Read the model definition and answer for the solid it produces. Units are mm, in the model's axes. A direction names the side the tool comes from. Coordinates: 2 decimals unless noted, no trailing zeros. Write each loop counter-clockwise with the first axis right and the second up, starting at its lowest first coordinate (ties: lowest second). Pieces come first, ordered by that corner, then holes.
Item 1: Section C-C (y = 6.5) is taken. Give the vertices of the cut face in (x, z), then the cut area to 3 significant figures.
Item 2: Determine the mould class of faces 1 (the face through (2.5, 1, -22.5)), 2 (the face through (2, -1, -5)), 3 (the face through (2, 0, -2)) for opening direction Z: released by +Z, released by -Z, zero draft, split by the parting line, or undercut.
Item 3: Each of these flat-tipped pins is pushed along its axis until it touches: P1, Ø2, axis at x = 1, z = -18, coming from the -Y side; P2, Ø1.6, axis at x = 3, y = -1, coming from the -Z side; P3, Ø1.5, axis at x = 2, z = -11, coming from the +Y side; P4, Ø2.5, axis at y = 7, z = -23, coming from the -X side. Where does it stop, or does it pass through?
Item 4: Section D-D (z = -23) is taken. Give the vertices of the cut face in (x, y).
Item 5: A tool of negligible diameter and unlimited length cuts with its end or side. For faces 4 (the face through (2, -2, -6)), 5 (the face through (0, 5, -13)), 6 (the face through (2, 0, -25)), 7 (the face through (0.76, 7.676, -25.146)), 8 (the face through (2, -1, -7)), from which of +Z, -Z, +X, -X, +Y, -Y can it reach the whole face along a straight path? Write none if from no direction.
Item 6: Section B-B (x = 0.55) is taken. Give the vertices of the cut face in (y, z), then the cut area to 3 significant figures.
Item 7: Section A-A (y = -0.5) is taken. Give the vertices of the cut face in (x, z).
Item 8: Straight lines are drawn through the part: probe 1 along Y at (x, z) = (3.3, -14); probe 2 along Z at (x, y) = (1.15, 0.75); probe 3 along Z at (x, y) = (1.1, 5). For each, find the intervals that lie inside material, in ascending order.
from build123d import *

# Parameters (mm, degrees)
BASE_W                    = 5
BASE_H                    = 26.5
BODY_DEPTH                = 11.5
F_6_0MM_MOTOR_D           = 6
F_3_0MM_BEARINGS_D        = 3
WEIGHT_SAVER_REACH        = 31.317
SKETCH9_W                 = 18.15
SKETCH9_H                 = 1.5
FILLET2_R                 = 3
FILLET1_R                 = 4
FILLET4_R                 = 4
FILLET5_R                 = 4
SKETCH10_W                = 5
SKETCH10_H                = 2
MOUNTING_DEPTH            = 2
MOUNTIN_UNDERCUT_REACH    = 31.317
F_4_0MM_DOWEL_HOLE2_D     = 4.5
F_4_0MM_DOWEL_HOLE2_DEPTH = 1.5


with BuildPart() as part:
    # base → body (new body)
    with BuildSketch(Plane(origin=(0, 0, 0), x_dir=(1, 0, 0), z_dir=(0, 1, 0))):
        with Locations((2.5, 13.25)):
            Rectangle(BASE_W, BASE_H)
    extrude(amount=BODY_DEPTH)

    # Ø6.0mm motor (through all)
    with Locations(Plane(origin=(5, 0, 0), x_dir=(0, 0, -1), z_dir=(1, 0, 0))):
        with Locations((5, 7)):
            Hole(F_6_0MM_MOTOR_D / 2)

    # Ø3.0mm bearings (through all)
    with Locations(Plane(origin=(5, 0, 0), x_dir=(0, 0, -1), z_dir=(1, 0, 0))):
        with Locations((14, 7), (23, 7)):
            Hole(F_3_0MM_BEARINGS_D / 2)

    # Sketch9 → weight_saver (cut, up to next)
    with BuildSketch(Plane(origin=(5, 0, 0), x_dir=(0, 0, -1), z_dir=(1, 0, 0)), mode=Mode.PRIVATE) as weight_saver_sk1:
        with Locations((17.425, 10.75)):
            Rectangle(SKETCH9_W, SKETCH9_H)
    weight_saver_tool1 = extrude(weight_saver_sk1.sketch, amount=-WEIGHT_SAVER_REACH, mode=Mode.PRIVATE) & part.part
    add(weight_saver_tool1.solids().sort_by_distance((5, 10.75, -17.425))[0], mode=Mode.SUBTRACT)

    # Fillet2
    fillet2_edges = [part.edges().sort_by_distance(p)[0] for p in [
        (2.5, 10, -26.5),
    ]]
    fillet(fillet2_edges, radius=FILLET2_R)

    # Fillet1
    fillet1_edges = [part.edges().sort_by_distance(p)[0] for p in [
        (2.5, 11.5, 0),
    ]]
    fillet(fillet1_edges, radius=FILLET1_R)

    # Fillet4
    # the kernel refuses this fillet: 4 mm, written as the material it adds along each edge
    with BuildSketch(Plane(origin=(5, 10, -8.35), x_dir=(0, 1, 0), z_dir=(-1, 0, 0))) as fillet4_piece_1:
        with BuildLine():
            CenterArc((4, 3.122498999), FILLET4_R, 180, 51.317812547)
            Line((0, 3.122498999), (-0.08, 3.122498999))
            Line((-0.08, 3.122498999), (-0.08, 0))
            Line((-0.08, 0), (0, -0.08))
            ThreePointArc((0, -0.08), (0.75, -0.08), (1.45, -0.06244998))
            Line((1.45, -0.06244998), (1.5, 0))
        make_face()
    extrude(amount=5)

    # Fillet5
    fillet5_edges = [part.edges().sort_by_distance(p)[0] for p in [
        (2.5, 11.5, -8.35),
    ]]
    fillet(fillet5_edges, radius=FILLET5_R)

    # Sketch10 → mounting (add)
    with BuildSketch(Plane.XZ):
        with Locations((2.5, -6)):
            Rectangle(SKETCH10_W, SKETCH10_H)
        with Locations((2.5, -20.5)):
            Rectangle(SKETCH10_W, SKETCH10_H)
    extrude(amount=MOUNTING_DEPTH)

    # mounting_undercut → mountin_undercut (cut, up to next)
    with BuildSketch(Plane(origin=(5, 0, 0), x_dir=(0, 0, -1), z_dir=(1, 0, 0)), mode=Mode.PRIVATE) as mountin_undercut_sk1:
        with BuildLine():
            Line((3, 0), (5, 0))
            ThreePointArc((5, 0), (4, 1), (3, 0))
        make_face()
    mountin_undercut_tool1 = extrude(mountin_undercut_sk1.sketch, amount=-MOUNTIN_UNDERCUT_REACH, mode=Mode.PRIVATE) & part.part
    # mounting_undercut → mountin_undercut (cut, up to next)
    with BuildSketch(Plane(origin=(5, 0, 0), x_dir=(0, 0, -1), z_dir=(1, 0, 0)), mode=Mode.PRIVATE) as mountin_undercut_sk2:
        with BuildLine():
            Line((7, 0), (9, 0))
            ThreePointArc((9, 0), (8, 1), (7, 0))
        make_face()
    mountin_undercut_tool2 = extrude(mountin_undercut_sk2.sketch, amount=-MOUNTIN_UNDERCUT_REACH, mode=Mode.PRIVATE) & part.part
    # mounting_undercut → mountin_undercut (cut, up to next)
    with BuildSketch(Plane(origin=(5, 0, 0), x_dir=(0, 0, -1), z_dir=(1, 0, 0)), mode=Mode.PRIVATE) as mountin_undercut_sk3:
        with BuildLine():
            Line((17.5, 0), (19.5, 0))
            ThreePointArc((19.5, 0), (18.5, 1), (17.5, 0))
        make_face()
    mountin_undercut_tool3 = extrude(mountin_undercut_sk3.sketch, amount=-MOUNTIN_UNDERCUT_REACH, mode=Mode.PRIVATE) & part.part
    # mounting_undercut → mountin_undercut (cut, up to next)
    with BuildSketch(Plane(origin=(5, 0, 0), x_dir=(0, 0, -1), z_dir=(1, 0, 0)), mode=Mode.PRIVATE) as mountin_undercut_sk4:
        with BuildLine():
            Line((21.5, 0), (23.5, 0))
            ThreePointArc((23.5, 0), (22.5, 1), (21.5, 0))
        make_face()
    mountin_undercut_tool4 = extrude(mountin_undercut_sk4.sketch, amount=-MOUNTIN_UNDERCUT_REACH, mode=Mode.PRIVATE) & part.part
    add(mountin_undercut_tool1.solids().sort_by_distance((5, 0.424413, -4))[0], mode=Mode.SUBTRACT)
    add(mountin_undercut_tool2.solids().sort_by_distance((5, 0.424413, -8))[0], mode=Mode.SUBTRACT)
    add(mountin_undercut_tool3.solids().sort_by_distance((5, 0.424413, -18.5))[0], mode=Mode.SUBTRACT)
    add(mountin_undercut_tool4.solids().sort_by_distance((5, 0.424413, -22.5))[0], mode=Mode.SUBTRACT)

    # Ø4.0mm Dowel Hole2
    with Locations(Plane.ZY):
        with Locations((-23, 7)):
            Hole(F_4_0MM_DOWEL_HOLE2_D / 2, depth=F_4_0MM_DOWEL_HOLE2_DEPTH)


solid = part.part
Established:
1. outline: (0, -26.5) - (5, -26.5) - (5, -24.41) - (1.5, -24.41) - (1.5, -25.19) - (0, -25.19) - close; (0, -20.81) - (1.5, -20.81) - (1.5, -21.59) - (5, -21.59) - (5, -15.41) - (0, -15.41) - close; (0, -12.59) - (5, -12.59) - (5, -7.96) - (0, -7.96) - close; (0, -2.04) - (5, -2.04) - (5, 0) - (0, 0) - close
1. area: 72.3 mm2
2. face 1: undercut
2. face 2: released by +Z
2. face 3: zero draft
3. P1: stops at y = 0
3. P2: stops at z = -21.5
3. P3: stops at y = 10.19
3. P4: passes through
4. outline: (0, 0.87) - (5, 0.87) - (5, 5.5) - (1.5, 5.5) - (1.5, 4.75) - (0, 4.75) - close; (0, 9.25) - (1.5, 9.25) - (1.5, 8.5) - (5, 8.5) - (5, 10) - (0, 10) - close
5. face 4: +Z, -Z, +X, -X, -Y
5. face 5: +Z, -Z, -X, +Y, -Y
5. face 6: -Z, +X, -X, -Y
5. face 7: -X
5. face 8: +X, -X, -Y
6. outline: (-2, -21.5) - (0, -21.5) arc R1 cw to (0, -23.5) - (0, -26.5) - (7, -26.5) arc R3 ccw to (10, -23.5) - (10, -11.47) arc R4 cw to (10.75, -9.14) arc R4 ccw to (11.5, -6.81) - (11.5, -4) arc R4 ccw to (7.5, 0) - (0, 0) - (0, -3) arc R1 cw to (0, -5) - (-2, -5) - (-2, -7) - (0, -7) arc R1 cw to (0, -9) - (0, -17.5) arc R1 cw to (0, -19.5) - (-2, -19.5) - close; hole circle Ø6 at (7, -5); hole circle Ø4.5 at (7, -23); hole circle Ø3 at (7, -14)
6. area: 224 mm2
7. outline: (0, -21.5) - (5, -21.5) - (5, -19.5) - (0, -19.5) - close; (0, -7) - (5, -7) - (5, -5) - (0, -5) - close
8. probe 1: y = 0 to 5.5, 8.5 to 10
8. probe 2: z = -26.5 to -23.16, -21.84 to -19.16, -17.84 to -8.66, -7.34 to -4.66, -3.34 to 0
8. probe 3: z = -26.5 to -24.03, -21.97 to -7.24, -2.76 to 0
